```python
from build123d import *

# Parameters (mm, degrees)
F1_DEPTH  = 3.5
F3_DEPTH  = 2
F4_R      = 1.55
F5_DEPTH  = 25
F7_DEPTH  = 25
F9_DEPTH  = 25
F10_R     = 1.55
F11_DEPTH = 2.5


with BuildPart() as f1:
    # F0 (on Top) → F1 (new body)
    with BuildSketch(Plane.XY):
        with BuildLine():
            Line((-5, 0), (-5, -3))
            Line((-5, -3), (2, -3))
            ThreePointArc((2, -3), (4.1213203436, -2.1213203436), (5, 0))
            Line((5, 0), (5, 3))
            Line((5, 3), (-2, 3))
            ThreePointArc((-2, 3), (-4.1213203436, 2.1213203436), (-5, 0))
        make_face()
    extrude(amount=F1_DEPTH)

    # F2 (on face) → F3 (join)
    with BuildSketch(Plane.XY.offset(3.5)):
        with BuildLine():
            Line((3, 0), (3, 3))
            Line((3, 3), (0, 3))
            ThreePointArc((0, 3), (-2.1213203436, 2.1213203436), (-3, 0))
            Line((-3, 0), (-3, -3))
            Line((-3, -3), (0, -3))
            ThreePointArc((0, -3), (2.1213203436, -2.1213203436), (3, 0))
        make_face()
    extrude(amount=F3_DEPTH)

    # F4 (on face) → F5 (cut)
    with BuildSketch(Plane.XY.offset(5.5)):
        Circle(F4_R)
    extrude(amount=-F5_DEPTH, mode=Mode.SUBTRACT)

    # F6 (on face) → F7 (cut)
    with BuildSketch(Plane.XZ.offset(3)):
        Polygon((-3.5, 0), (-5, 1.75), (-5, 0), align=None)
    extrude(amount=-F7_DEPTH, mode=Mode.SUBTRACT)

    # F8 (on face) → F9 (cut)
    with BuildSketch(Plane(origin=(0, 3, 0), x_dir=(-1, 0, 0), z_dir=(0, 1, 0))):
        Polygon((-5, 0), (-3.5, 0), (-5, 1.75), align=None)
    extrude(amount=-F9_DEPTH, mode=Mode.SUBTRACT)

    # F10 (on face) → F11 (cut)
    with BuildSketch(Plane(origin=(0, 0, 0), x_dir=(1, 0, 0), z_dir=(0, 0, -1))):
        Polygon((1.8021214103, -3), (3.5, -0.128752487), (3.5, 0.0591513549), (1.8427445262, 3), (-1.8021214103, 3), (-3.5, 0.128752487), (-3.5, -0.0591513549), (-1.8427445262, -3), align=None)
        Circle(F10_R, mode=Mode.SUBTRACT)
    extrude(amount=-F11_DEPTH, mode=Mode.SUBTRACT)


solid = f1.part
```
The listing builds one solid part. Answer for the finished solid, in the listing's coordinates (mm). A direction names the side the tool comes from. Coordinates: 2 decimals unless noted, no trailing zeros. Write each loop counter-clockwise with the first axis right and the second up, starting at its lowest first coordinate (ties: lowest second). Pieces come first, ordered by that corner, then holes. Notation, with made-up numbers: (-32.75, 54.5) -> (4.25, 54.5) arc R24 cw to (4.25, 74.5) -> close; hole circle Ø2 at (69.25, 87). An arc over 180 degrees is marked (long way). Write each question's results on one line, items separated by ' | '. Start each with the question number.
1) Straight lines are drawn through the part: probe 1 along Y at (x, z) = (0, 3.2); probe 2 along Z at (x, y) = (-2.5, -1.75); probe 3 along X at (y, z) = (-0.75, 1.55). For each, find the intervals that lie inside material, in ascending order.
2) A cutting plane is placed at B-B (z = 3.75). Determine the outline of the cut face in (x, y).
3) A cutting plane is placed at A-A (z = 0.35). Determine the outline of the cut face in (x, y), then the cut area to 3 significant figures.
4) A tool of negligible diameter and unlimited length cuts with its end or side. For faces 1 (the flat face through (2.64, 1.58, 1.23)), 2 (the flat face through (5, 1, 3)), 3 (the flat face through (3, 1, 4)), 4 (the flat face through (-3, -1, 4)), from which of +Z, -Z, +X, -X, +Y, -Y can it reach the whole face along a straight path? Write none if from no direction.
5) Flat-ended cylindrical pins translate along their axes: pin 1 Ø3 at (x, z) = (2, 4) entering from -Y; pin 2 Ø1 at (y, z) = (-1, 4.5) entering from -X; pin 3 Ø0.6 at (y, z) = (1.5, 4) entering from +X; pin 4 Ø1.5 at (y, z) = (2, 3) entering from -X. Find the tip coordinate at first contact, or state that the pin passes through.
6) A cutting plane is placed at C-C (x = -0.75). Determine the outline of the cut face in (y, z), then the cut area to 3 significant figures.
7) A cutting plane is placed at D-D (z = 2.35). Determine the outline of the cut face in (x, y), then the cut area to 3 significant figures.
8) For a pull along Y with two mould halves and no side action, classify faces 5 (the flat face through (3, 2, 0)), 6 (the cylindrical face through (-2.1, 2.14, 4.49)), 7 (the flat face through (-2.683, 1.509, 1.232)) as +Y half, -Y half, draft (parallel to the pull), parting line (faces both ways), or undercut.
Values follow:
1) probe 1: -3 to -1.55, 1.55 to 3 | probe 2: 2.5 to 5.5 | probe 3: -4.83 to -3.13, 3.11 to 4.83
2) outline: (-3, -3) -> (0, -3) arc R3 ccw to (3, 0) -> (3, 3) -> (0, 3) arc R3 ccw to (-3, 0) -> close; hole circle Ø3.1 at (0, 0)
3) outline: (-3.8, -3) -> (-1.8, -3) -> (-3.5, -0.13) -> (-3.5, 0.06) -> (-1.84, 3) -> (-2, 3) arc R3 ccw to (-3.8, 2.4) -> close; (1.8, 3) -> (3.5, 0.13) -> (3.5, -0.06) -> (1.84, -3) -> (2, -3) arc R3 ccw to (3.8, -2.4) -> (3.8, 3) -> close | area: 12.7 mm²
4) face 1: -Z | face 2: +Z, -Z, +X, +Y, -Y | face 3: +Z, +X, +Y, -Y | face 4: +Z, -X, +Y, -Y
5) pin 1: y = -3 | pin 2: x = -3 | pin 3: x = 3 | pin 4: x = -4.73
6) outline: (-3, 2.5) -> (-1.36, 2.5) -> (-1.36, 5.5) -> (-3, 5.5) -> close; (1.36, 2.5) -> (3, 2.5) -> (3, 3.5) -> (2.9, 3.5) -> (2.9, 5.5) -> (1.36, 5.5) -> close | area: 9.67 mm²
7) outline: (-5, -3) -> (-1.8, -3) -> (-3.5, -0.13) -> (-3.5, 0.06) -> (-1.84, 3) -> (-2, 3) arc R3 ccw to (-5, 0) -> close; (1.8, 3) -> (3.5, 0.13) -> (3.5, -0.06) -> (1.84, -3) -> (2, -3) arc R3 ccw to (5, 0) -> (5, 3) -> close | area: 23.9 mm²
8) face 5: draft | face 6: +Y half | face 7: undercut
